Could you check a few things on this model? Use its own coordinates, in mm. A direction names the side the tool comes from. Coordinates: 2 decimals unless noted, no trailing zeros. Order: outer loops, then holes, each group sorted by start corner. A loop starts at its lowest first (then second) coordinate and runs counter-clockwise, first axis right, second up. Notation, with made-up numbers: (31, 89.5) - (68, 89.5) arc R23 cw to (68, 103.5) - close; hole circle Ø5 at (22.5, -36). An arc over 180 degrees is marked (long way). Answer as CSV lines item,"result". Start each with the question number.
1. I need wall thicknesses on probe 1 along X at (y, z) = (3.25, -8); probe 2 along Z at (x, y) = (-12, 5.5). Which ranges of each line are inside material? Lowest first, please.
2. For pin 1 (5.5 mm diameter, centred on x = -14, z = 7, fed in from -Y); pin 2 (1.5 mm diameter, centred on x = -10.5, y = 5, fed in from +Z); pin 3 (2 mm diameter, centred on x = -9.5, z = 6.5, fed in from +Y), each with a flat end and sliding along its axis, tell me the tip position at first contact or that it passes through.
3. I want a section at D-D, the plane z = 3.75. List the corners of the cut face in (x, y) for me.
4. For faces 1 (the face through (-12, 5, 10)), 2 (the face through (-12, 3.5, 7)), 3 (the face through (-12, 6.5, 7)), 4 (the face through (-12, 5, 5)), which set-ups out of +Z, -Z, +X, -X, +Y, -Y let a thin tool reach every point of the face, with its end or its side?
5. I want a section at C-C, the plane x = -13. List the corners of the cut face in (y, z) for me.
6. I want a section at A-A, the plane z = 6.75. List the corners of the cut face in (x, y) for me.
7. I want a section at B-B, the plane y = 4.75. List the corners of the cut face in (x, z) for me, and give its area (3 significant figures).
from build123d import *

# Parameters (mm, degrees)
F0_W     = 15
F0_H     = 30
F1_DEPTH = 10
F2_W     = 3
F2_H     = 5
F3_DEPTH = 10


with BuildPart() as f1:
    # F0 (on Front) → F1 (new body)
    with BuildSketch(Plane.XZ):
        Rectangle(F0_W, F0_H)
    extrude(amount=-F1_DEPTH)

    # F2 (on face) → F3 (join)
    with BuildSketch(Plane(origin=(-7.5, 0, 0), x_dir=(0, -1, 0), z_dir=(-1, 0, 0))):
        with Locations((-5, 7.5)):
            Rectangle(F2_W, F2_H)
    extrude(amount=F3_DEPTH)


solid = f1.part
Solved:
1,probe 1,"x = -7.5 to 7.5"
1,probe 2,"z = 5 to 10"
2,pin 1,"stops at y = 3.5"
2,pin 2,"stops at z = 10"
2,pin 3,"stops at y = 6.5"
3,outline,"(-7.5, 0) - (7.5, 0) - (7.5, 10) - (-7.5, 10) - close"
4,face 1,"+Z, -X, +Y, -Y"
4,face 2,"+Z, -Z, -X, -Y"
4,face 3,"+Z, -Z, -X, +Y"
4,face 4,"-Z, -X, +Y, -Y"
5,outline,"(3.5, 5) - (6.5, 5) - (6.5, 10) - (3.5, 10) - close"
6,outline,"(-17.5, 3.5) - (-7.5, 3.5) - (-7.5, 0) - (7.5, 0) - (7.5, 10) - (-7.5, 10) - (-7.5, 6.5) - (-17.5, 6.5) - close"
7,outline,"(-17.5, 5) - (-7.5, 5) - (-7.5, -15) - (7.5, -15) - (7.5, 15) - (-7.5, 15) - (-7.5, 10) - (-17.5, 10) - close"
7,area,"500 mm2"
